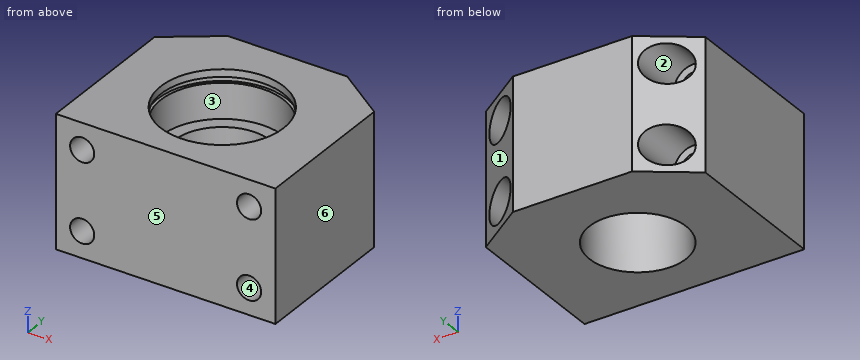
```python
from build123d import *

# Parameters (mm, degrees)
SZKIC1_W                                             = 50
SZKIC1_H                                             = 30
DODANIE_WYCI_GNI_CIE1_DEPTH                          = 42
SZKIC3_R                                             = 11
WYTNIJ_WYCI_GNI_CIE2_DEPTH                           = 58.349803836
SZKIC4_R                                             = 14
WYTNIJ_WYCI_GNI_CIE3_DEPTH                           = 11
POG_BIENIE_WALCOWE_POD_M5_WKR_T_DO_CZ_CI_D           = 5.5
POG_BIENIE_WALCOWE_POD_M5_WKR_T_DO_CZ_CI_CBORE_D     = 9
POG_BIENIE_WALCOWE_POD_M5_WKR_T_DO_CZ_CI_CBORE_DEPTH = 13
SZKIC5_W                                             = 1.3
SZKIC5_H                                             = 0.7
WYTNIJ_WYCI_GNI_CIE5_DEPTH                           = 58.349803836


with BuildPart() as part:
    # Szkic1 → Dodanie-wyciągnięcie1 (new body)
    with BuildSketch(Plane(origin=(0, 0, 0), x_dir=(1, 0, 0), z_dir=(0, 1, 0))):
        Rectangle(SZKIC1_W, SZKIC1_H)
    extrude(amount=DODANIE_WYCI_GNI_CIE1_DEPTH)

    # Szkic3 → Wytnij-wyciągnięcie2 (cut, through all)
    with BuildSketch(Plane.XY.offset(15)):
        with Locations((0, 19.5)):
            Circle(SZKIC3_R)
    extrude(amount=-WYTNIJ_WYCI_GNI_CIE2_DEPTH, mode=Mode.SUBTRACT)

    # Szkic4 → Wytnij-wyciągnięcie3 (cut)
    with BuildSketch(Plane.XY.offset(15)):
        with Locations((0, 19.5)):
            Circle(SZKIC4_R)
    extrude(amount=-WYTNIJ_WYCI_GNI_CIE3_DEPTH, mode=Mode.SUBTRACT)

    # Pogłębienie walcowe pod M5 Wkręt do części metalowych z łbem sześciokątnym1 (through all)
    with Locations(Plane(origin=(0, 42, 0), x_dir=(1, 0, 0), z_dir=(0, 1, 0))):
        with Locations((19, 9), (19, -9), (-19, -9), (-19, 9)):
            CounterBoreHole(POG_BIENIE_WALCOWE_POD_M5_WKR_T_DO_CZ_CI_D / 2, POG_BIENIE_WALCOWE_POD_M5_WKR_T_DO_CZ_CI_CBORE_D / 2, POG_BIENIE_WALCOWE_POD_M5_WKR_T_DO_CZ_CI_CBORE_DEPTH)

    # Szkic5 → Wycięcie-obrót1 (revolve, cut)
    with BuildSketch(Plane(origin=(0, 0, 0), x_dir=(0, 0, -1), z_dir=(1, 0, 0)), mode=Mode.PRIVATE) as wyci_cie_obr_t1_sk:
        with Locations((-12.65, 5.15)):
            Rectangle(SZKIC5_W, SZKIC5_H)
    revolve(wyci_cie_obr_t1_sk.sketch.rotate(Axis((0, 19.5, 9.294649117), (0, 0, 1)), 90), axis=Axis((0, 19.5, 9.294649117), (0, 0, 1)), mode=Mode.SUBTRACT)

    # Szkic9 → Wytnij-wyciągnięcie5 (cut, through all)
    with BuildSketch(Plane.XY.offset(15)):
        Polygon((-25, 34), (-13.574815946, 42), (-25, 42), align=None)
        Polygon((25, 42), (13.574815946, 42), (25, 34), align=None)
    extrude(amount=-WYTNIJ_WYCI_GNI_CIE5_DEPTH, mode=Mode.SUBTRACT)


solid = part.part
```
Geometry check sheet. Reference: the model listing, model coordinates, mm. Face numbers are marked on the shaded views. A direction names the side the tool comes from. Give positions to 0.01 mm unless a question says otherwise; leave off trailing zeros. Loops run counter-clockwise (first coordinate to the right, second up) from the corner with the lowest first, then second, coordinate; pieces in that order, holes last. Notation, with made-up numbers: M 31.5,78 L 59.5,78 A33 ccw 59.5,109 Z; hole C 66.25,41 d9. An arc over 180 degrees is marked long. Write item = value, one per line. Start each with the question number.
1. Section check A-A, the plane y = 19.5. Enter the section's corners in (x, z), plus the area to 3 significant figures.
2. Draft check along X on the marked faces 4, 5 and 6. Enter one of: +X half, -X half, draft (parallel to the pull), parting line (faces both ways), or undercut.
3. Section check C-C, the plane x = 0. Enter the section's corners in (y, z).
4. Thickness scan on probe 1 along Z at (x, y) = (19, 34); probe 2 along Z at (x, y) = (-19, 20.5); probe 3 along Y at (x, z) = (0, 13). Record the ranges inside material, lowest first.
5. Go/stop test with flat-tipped pins: P1, Ø4, axis at x = 17.5, z = -8.5, coming from the +Y side; P2, Ø25, axis at x = 0, y = 19.5, coming from the +Z side; P3, Ø1.5, axis at x = 4, z = 10.5, coming from the -Y side; P4, Ø7, axis at x = 17.5, z = 7, coming from the +Y side. Record where each tip stops, or that it passes through.
6. Section check B-B, the plane z = -1. Enter the section's corners in (x, y).
7. Section check D-D, the plane z = -9. Enter the section's corners in (x, y), plus the area to 3 significant figures.
8. Tool access check on the marked faces 1, 2 and 3. Record the directions out of +Z, -Z, +X, -X, +Y, -Y that give a thin tool (end or side, any length) a straight path to the whole face; none if there is none.
Values follow:
q1.outline = M -25,-15 L -11,-15 L -11,4 L -14,4 L -14,12 L -14.7,12 L -14.7,13.3 L -14,13.3 L -14,15 L -25,15 Z; M 11,-15 L 25,-15 L 25,15 L 14,15 L 14,13.3 L 14.7,13.3 L 14.7,12 L 14,12 L 14,4 L 11,4 Z; hole C -19,-9 d5.5; hole C -19,9 d5.5; hole C 19,-9 d5.5; hole C 19,9 d5.5
q1.area = 677 mm^2
q2.face_4 = undercut
q2.face_5 = draft
q2.face_6 = +X half
q3.outline = M 0,-15 L 8.5,-15 L 8.5,4 L 5.5,4 L 5.5,12 L 4.8,12 L 4.8,13.3 L 5.5,13.3 L 5.5,15 L 0,15 Z; M 30.5,-15 L 42,-15 L 42,15 L 33.5,15 L 33.5,13.3 L 34.2,13.3 L 34.2,12 L 33.5,12 L 33.5,4 L 30.5,4 Z
q4.probe_1 = -15 to -13.5, -4.5 to 4.5, 13.5 to 15
q4.probe_2 = -15 to -11.75, -6.25 to 6.25, 11.75 to 15
q4.probe_3 = 0 to 4.8, 34.2 to 42
q5.P1 = 29
q5.P2 = 4
q5.P3 = 0
q5.P4 = 41.7
q6.outline = M -25,0 L 25,0 L 25,34 L 13.57,42 L -13.57,42 L -25,34 Z; hole C 0,19.5 d22
q7.outline = M -25,0 L -21.75,0 L -21.75,29 L -23.5,29 L -23.5,35.05 L -25,34 Z; M -16.25,0 L 16.25,0 L 16.25,29 L 14.5,29 L 14.5,41.35 L 13.57,42 L -13.57,42 L -14.5,41.35 L -14.5,29 L -16.25,29 Z; M 21.75,0 L 25,0 L 25,34 L 23.5,35.05 L 23.5,29 L 21.75,29 Z; hole C 0,19.5 d22
q7.area = 1,140 mm^2
q8.face_1 = +Z, -Z, +X, +Y
q8.face_2 = +Y
q8.face_3 = +Z
